Source: CAD feature listing. Evaluate the final solid. Frame: model axes, mm. A direction names the side the tool comes from. Round coordinates to 2 decimals unless told otherwise and drop trailing zeros. Order: outer loops, then holes, each group sorted by start corner. A loop starts at its lowest first (then second) coordinate and runs counter-clockwise, first axis right, second up. Notation, with made-up numbers: (-11, 20) -> (17, 20) arc R16 cw to (17, 42) -> close; hole circle Ø11 at (78.25, -15.5). An arc over 180 degrees is marked (long way). Answer as CSV lines item,"result". Start each with the question number.
(1) Pull-direction query (X, two-part tool) for faces 6 (the cylindrical face through (-6.45, 2.71, 0.14)), 7 (the cylindrical face through (1.32, 3.49, -0.29)), 8 (the flat face through (37, 2, -15)); classes: +X half, -X half, draft (parallel to the pull), parting line (faces both ways), or undercut.
(2) Section query B-B (x = 32.5). Output: boundary loops of the cut face in (y, z).
(3) Section query A-A (z = -0.5). Count the separate pieces of the cut face and the enclosed holes in it, plus the area to 3 significant figures.
(4) Section query D-D (x = 26.5). Output: boundary loops of the cut face in (y, z), plus the area to 3 significant figures.
(5) Line query: line 1 along Z through (x, y) = (0, 4.5); line 2 along Z through (x, y) = (0, 3.35); line 3 along Y through (x, z) = (30.5, -6). Output: solid intervals per line, ascending. Write a range as from..to.
(6) Set-up query: faces 1 (the flat face through (11.32, 2.1, -5.522)), 2 (the cylindrical face through (-2.947, 1.479, 0.13)), 3 (the cylindrical face through (25, 2, 0)), 4 (the flat face through (28, 4, -5)), 5 (the flat face through (21, 0, -2)). Return all of +Z, -Z, +X, -X, +Y, -Y with unobstructed straight access to the full face (end or side cutting, diameter ignored); none if empty.
(7) Contact query for flat-ended pins moving along their axis: P1, Ø12, axis at x = 34, z = -0.5, coming from the +Y side; P2, Ø3, axis at x = 27.5, y = 4.5, coming from the -Z side; P3, Ø2, axis at x = 14, y = 2, coming from the +Z side. Output: stop coordinate, or through.
(8) Section query C-C (y = 1.65). Output: boundary loops of the cut face in (x, z).
Autodesk Inventor part; units mm, degrees
ref_plane "YZ Plane" through (0, 0, 0) normal (1, 0, 0) x (0, 1, 0)
ref_plane "XZ Plane" through (0, 0, 0) normal (0, 1, 0) x (-1, 0, 0)
ref_plane "XY Plane" through (0, 0, 0) normal (0, 0, 1) x (1, 0, 0)
sketch "Sketch1" plane through (0, 0, 0) normal (0, 1, 0) x (-1, 0, 0)
  circle A0 centre (0, 0) radius 6.45
  circle A1 centre (0, 0) radius 5.657
  circle A2 centre (0, 0) radius 2.85
  line L0 (0, 0) -> (-36, 0) construction
  circle A3 centre (-36, 0) radius 3.5
  line L1 (0, -6.45) -> (-36, -3.5)
  line L2 (0, 6.45) -> (-36.2847, 3.4884)
  dimension "d0" = 12.9
  dimension "d1" = 11.314
  dimension "d2" = 5.7
  dimension "d3" = 36
  dimension "d4" = 7
extrude "Extrusion1" add sketch "Sketch1" along normal blind 4 contours A0 L1 L2 | A0 L1 A3 L2 | A3 | A1 | A2
sketch "Sketch2" plane through (0, 4, 0) normal (0, 1, 0) x (1, 0, 0)
  circle A0 centre (0, 0) radius 6.45
  line L0 (36, 3.5) -> (0, 6.45)
  line L1 (0, -6.45) -> (36.2847, -3.4884)
  arc A1 (0, 6.45) -> (0, -6.45) centre (0, 0) ccw
  line L2 (9.9188, -5.6404) -> (9.9188, 5.6372)
  line L3 (9.9188, 5.6372) -> (0, 6.45)
  line L4 (0, -6.45) -> (9.9188, -5.6404)
  dimension "d7" = 12.9
extrude "Extrusion2" add sketch "Sketch2" along normal blind 1.5 contours L0 A0 L1 | L0 L2 L1 A0
fillet "Fillet1" radius 10 1 edges at (9.9188, 5.5, 0.0016)
sketch "Sketch3" plane through (0, 5.5, 0) normal (0, 1, 0) x (1, 0, 0)
  circle A0 centre (0, 0) radius 5.657
  dimension "d11" = 11.314
extrude "Extrusion3" cut sketch "Sketch3" against normal blind 1.5
sketch "Sketch4" plane through (0, 4, 0) normal (0, 1, 0) x (1, 0, 0)
  circle A0 centre (0, 0) radius 2.9
  dimension "d14" = 5.8
sketch "Sketch5" plane through (0, 0, 0) normal (0, -1, 0) x (1, 0, 0)
  circle A0 centre (0, 0) radius 2.95
  dimension "d15" = 5.9
extrude "Extrusion4" cut sketch "Sketch5" against normal blind 3
sketch "Sketch6" plane through (0, 4, 0) normal (0, 1, 0) x (1, 0, 0)
  circle A0 centre (0, 0) radius 1.35
  dimension "d18" = 2.7
hole "Hole1" at (0, 4, 0) direction (0, -1, 0) diameter 2.7 end through all
sketch "Sketch7" plane through (0, 0, 0) normal (0, -1, 0) x (1, 0, 0)
  point P0 (0, 0)
sketch "Sketch8" plane through (0, 4, 0) normal (0, 1, 0) x (1, 0, 0)
  line L0 (9.9188, 5.6372) -> (9.9188, -5.6404) construction
  line L1 (9.9188, -0.0016) -> (39.5, -0.0016) construction
  arc A0 (36.2847, -3.4884) -> (36, 3.5) centre (36, 0) ccw construction
  line L2 (32.5, -0.0016) -> (26.5, -0.0016) construction
  circle A1 centre (26.5, -0.0016) radius 1.5 construction
  line L3 (26.5, -0.0016) -> (20.5, -0.0016) construction
  circle A2 centre (20.5, -0.0016) radius 1.5 construction
  circle A3 centre (32.5, -0.0016) radius 1.5 construction
  circle A4 centre (32.5, -0.0016) radius 1.5 construction
  circle A5 centre (32.5, -0.0016) radius 1.5
  circle A6 centre (26.5, -0.0016) radius 1.5
  circle A7 centre (20.5, -0.0016) radius 1.5
  point P0 (0, 0)
  dimension "d27" = 6
  dimension "d28" = 3
  dimension "d29" = 6
  dimension "d30" = 3
  dimension "d31" = 3
  dimension "d32" = 3
  dimension "d33" = 3
  dimension "d34" = 3
hole "Hole2" at (20.5, 4, 0.0016) at (26.5, 4, 0.0016) at (32.5, 4, 0.0016) direction (0, -1, 0) diameter 3 end through all
sketch "Sketch9" plane through (0, 4, 0) normal (0, 1, 0) x (1, 0, 0)
  arc A0 (36.2847, -3.4884) -> (36, 3.5) centre (36, 0) ccw
  line L0 (39.5, 0) -> (39.5, 15)
  line L1 (39.5, 15) -> (22.9619, 15)
  line L2 (22.9619, 15) -> (22.9619, 4.5684)
  line L3 (36, 3.5) -> (0, 6.45)
  point P0 (0, 0)
  dimension "d46" = 15
extrude "Extrusion5" add sketch "Sketch9" against normal blind 4
sketch "Sketch10" plane through (0, 4, 0) normal (0, 1, 0) x (1, 0, 0)
  line L0 (39.5, 15) -> (22.9619, 15)
  line L1 (22.9619, 15) -> (39.5, 15)
  line L2 (22.9619, 15) -> (39.5, 15)
  arc A0 (23.6935, 15) -> (35.6591, 15) centre (29.6763, 28.5077) ccw
  point P0 (0, 0)
extrude "Extrusion6" [suppressed]
sketch "Sketch11" plane through (0, 4, 0) normal (0, 1, 0) x (1, 0, 0)
  circle A0 centre (20.5, -0.0016) radius 1.5 construction
  line L0 (19, -0.0016) -> (16, -0.0016) construction
  circle A1 centre (14.4602, -0.0016) radius 1.5 construction
  circle A2 centre (14.4602, -0.0016) radius 1.5
  point P0 (0, 0)
  dimension "d47" = 3
  dimension "d48" = 3
hole "Hole3" at (14.4602, 4, 0.0016) direction (0, -1, 0) diameter 3 end through all
sketch "Sketch12" plane through (0, 4, 0) normal (0, 1, 0) x (1, 0, 0)
  line L0 (39.5, 15) -> (22.9619, 15)
  line L1 (22.9619, 15) -> (39.5, 15)
  arc A0 (22.9619, 15) -> (34.5413, 15) centre (28.7516, 24.0306) ccw
  point P0 (0, 0)
extrude "Extrusion7" cut sketch "Sketch12" against normal blind 4
properties part number "servo_arm_3"
Answer block:
1,face 6,"-X half"
1,face 7,"undercut"
1,face 8,"draft"
2,outline,"(0, -13.98) -> (4, -13.98) -> (4, -1.5) -> (0, -1.5) -> close; (0, 1.5) -> (4, 1.5) -> (4, 3.8) -> (0, 3.8) -> close"
3,separate pieces,"6"
3,enclosed holes,"0"
3,area,"124 mm2"
4,outline,"(0, -13.54) -> (4, -13.54) -> (4, -1.5) -> (0, -1.5) -> close; (0, 1.5) -> (4, 1.5) -> (4, 4.29) -> (0, 4.29) -> close"
4,area,"59.3 mm2"
5,line 1,"-6.45..-5.66, 5.66..6.45"
5,line 2,"-6.45..-1.35, 1.35..6.45"
5,line 3,"0..4"
6,face 1,"-Z, +Y, -Y"
6,face 2,"-Y"
6,face 3,"+Y, -Y"
6,face 4,"+Z, -Z, +X, +Y"
6,face 5,"+Z, -Z, +X, -X, -Y"
7,P1,"y = 4"
7,P2,"z = -13.64"
7,P3,"z = 5.39"
8,outline,"(0, -6.45) -> (22.96, -4.57) -> (22.96, -15) arc R10.73 cw to (34.54, -15) -> (39.5, -15) -> (39.5, 0) arc R3.5 ccw to (36.28, 3.49) -> (0, 6.45) arc R6.45 ccw to start; hole circle Ø5.9 at (0, 0); hole circle Ø3 at (14.46, 0); hole circle Ø3 at (20.5, 0); hole circle Ø3 at (26.5, 0); hole circle Ø3 at (32.5, 0)"
